```python
from build123d import *

# Parameters (mm, degrees)
BOSS_EXTRUDE1_DEPTH     = 50
CUT_EXTRUDE1_DEPTH      = 51.970579749
SKETCH4_W               = 15
SKETCH4_H               = 10
BOSS_EXTRUDE2_DEPTH     = 12
SKETCH5_R               = 2.5
CUT_EXTRUDE2_DEPTH      = 10
CUT_EXTRUDE3_REACH      = 38.892
CUT_EXTRUDE3_END_RADIUS = 2.5
SKETCH6_R               = 2.25


with BuildPart() as part:
    # Sketch2 → Boss-Extrude1 (new body)
    with BuildSketch(Plane(origin=(0, 0, 0), x_dir=(0, 0, -1), z_dir=(1, 0, 0))):
        Polygon((0, -7), (0, 7), (10, 7), (10, 5), (3, 5), (3, -5), (10, -5), (10, -7), align=None)
    extrude(amount=BOSS_EXTRUDE1_DEPTH)

    # Sketch3 → Cut-Extrude1 (cut, through all)
    with BuildSketch(Plane(origin=(0, 0, -3), x_dir=(-1, 0, 0), z_dir=(0, 0, -1))):
        with BuildLine():
            Line((-41, 3), (-9, 3))
            ThreePointArc((-9, 3), (-6, 0), (-9, -3))
            Line((-9, -3), (-41, -3))
            ThreePointArc((-41, -3), (-44, 0), (-41, 3))
        make_face()
    extrude(amount=-CUT_EXTRUDE1_DEPTH, mode=Mode.SUBTRACT)

    # Sketch4 → Boss-Extrude2 (add)
    with BuildSketch(Plane(origin=(0, 7, 0), x_dir=(1, 0, 0), z_dir=(0, 1, 0))):
        with Locations((22.5, 5)):
            Rectangle(SKETCH4_W, SKETCH4_H)
    extrude(amount=BOSS_EXTRUDE2_DEPTH)

    # Sketch5 → Cut-Extrude2 (cut)
    with BuildSketch(Plane(origin=(0, 19, 0), x_dir=(1, 0, 0), z_dir=(0, 1, 0))):
        with Locations(Location((20, 5, 0), (0, 0, 270))):
            Circle(SKETCH5_R)
    extrude(amount=-CUT_EXTRUDE2_DEPTH, mode=Mode.SUBTRACT)

    # Cut-Extrude3: up to this cylinder (the profile starts outside it)
    cut_extrude3_end = Plane(origin=(20, 13, -5), z_dir=(0, 1, 0)) * Cylinder(CUT_EXTRUDE3_END_RADIUS, 83.784, mode=Mode.PRIVATE)
    # Sketch6 → Cut-Extrude3 (cut, up to the surface)
    with BuildSketch(Plane(origin=(30, 0, 0), x_dir=(0, 0, -1), z_dir=(1, 0, 0)), mode=Mode.PRIVATE) as cut_extrude3_sk1:
        with Locations((5, 13)):
            Circle(SKETCH6_R)
    cut_extrude3_tool1 = extrude(cut_extrude3_sk1.sketch, amount=-CUT_EXTRUDE3_REACH, mode=Mode.PRIVATE) - cut_extrude3_end
    add(cut_extrude3_tool1.solids().sort_by_distance((30, 13, -5))[0], mode=Mode.SUBTRACT)


solid = part.part
```
Geometry: final body of the model. Coordinates: model frame, mm. A direction names the side the tool comes from. Coordinates: 2 decimals unless noted, no trailing zeros. Order: outer loops, then holes, each group sorted by start corner. A loop starts at its lowest first (then second) coordinate and runs counter-clockwise, first axis right, second up.
Item 1: Material intervals for line 1 along Y through (x, z) = (26.5, -5); line 2 along Z through (x, y) = (28, 13); line 3 along X through (y, z) = (16, -5), sorted ascending.
Answer:
line 1: y = -7 to -5, 5 to 10.75, 15.25 to 19
line 2: z = -10 to -7.25, -2.75 to 0
line 3: x = 15 to 17.5, 22.5 to 30
Item 2: Section query C-C (y = 0). Output: boundary loops of the cut face in (x, z).
Answer:
outline: (0, -3) - (6, -3) - (6, 0) - (0, 0) - close; (44, -3) - (50, -3) - (50, 0) - (44, 0) - close
Item 3: Section query A-A (x = 33.5). Output: boundary loops of the cut face in (y, z).
Answer:
outline: (-7, -10) - (-5, -10) - (-5, -3) - (-3, -3) - (-3, 0) - (-7, 0) - close; (3, -3) - (5, -3) - (5, -10) - (7, -10) - (7, 0) - (3, 0) - close
Item 4: Draft query along X for faces 1 (the face through (25, -7, -5)), 2 (the face through (25, 3, -2)), 3 (the face through (0, 0.1, -2.8)). Return one class per face: released by +X, released by -X, zero draft, split by the parting line, or undercut.
Answer:
face 1: zero draft
face 2: undercut
face 3: released by -X
Item 5: Section query D-D (x = 18). Output: boundary loops of the cut face in (y, z).
Answer:
outline: (-7, -10) - (-5, -10) - (-5, -3) - (-3, -3) - (-3, 0) - (-7, 0) - close; (3, -3) - (5, -3) - (5, -10) - (19, -10) - (19, -6.5) - (9, -6.5) - (9, -3.5) - (19, -3.5) - (19, 0) - (3, 0) - close
Item 6: Section query B-B (z = -5). Output: boundary loops of the cut face in (x, y).
Answer:
outline: (0, -7) - (50, -7) - (50, -5) - (0, -5) - close; (0, 5) - (50, 5) - (50, 7) - (30, 7) - (30, 10.75) - (22.5, 10.75) - (22.5, 9) - (17.5, 9) - (17.5, 19) - (15, 19) - (15, 7) - (0, 7) - close; (22.5, 15.25) - (30, 15.25) - (30, 19) - (22.5, 19) - close
Item 7: Access query for faces 4 (the face through (24.6, 3.4, -3)), 5 (the face through (17.78, 14.07, -3.85)), 6 (the face through (25.607, 13.676, -7.146)), 7 (the face through (25, -3, -2)). Directions: +Z, -Z, +X, -X, +Y, -Y. A direction counts if a zero-diameter tool reaches every point of the face in a straight line with its end or side. Return the directions, or none.
Answer:
face 4: -Z, +X, -X
face 5: +Y
face 6: +X
face 7: +Z, -Z
Item 8: Contact query for flat-ended pins moving along their axis: P1, Ø5, axis at y = 13.5, z = -6.5, coming from the -X side; P2, Ø4, axis at x = 40.5, z = -7, coming from the +Y side; P3, Ø6, axis at y = 13, z = -5, coming from the +X side. Output: stop coordinate, or through.
Answer:
P1: stops at x = 15
P2: stops at y = 7
P3: stops at x = 30
